Could you check a few things on this model? Use its own coordinates, in mm. A direction names the side the tool comes from. Round coordinates to 2 decimals unless told otherwise and drop trailing zeros. Loops run counter-clockwise (first coordinate to the right, second up) from the corner with the lowest first, then second, coordinate; pieces in that order, holes last. Notation, with made-up numbers: (10, 41) -> (51, 41) arc R27 ccw to (51, 80) -> close; hole circle Ø8 at (-19.5, 84.25). An arc over 180 degrees is marked (long way). Write each question's results on one line, items separated by ' | '. Start each with the question number.
1) Imagine slicing it at A-A, the plane x = 2.5. List the corners of the cut face in (y, z) for me.
2) For P1, Ø3, axis at y = 0, z = 2.5, coming from the +X side, with a flat end and sliding along its axis, tell me the tip position at first contact or that it passes through.
3) If I drill on probe 1 along X at (y, z) = (14.7, 0); probe 2 along Z at (x, y) = (2.5, 15.35); probe 3 along Y at (x, z) = (-1.75, 1.25), over which ranges is the centre line in solid material (lowest first)?
4) Which directions (+Z, -Z, +X, -X, +Y, -Y) give clear straight access to the entire face, cutting with the end or side of a thin tool? Please do faces 1 (the flat face through (0, 14, 0)), 2 (the cylindrical face through (0.35, -15.48, -0.09)).
5) We'd pull the mould along Z, two halves only. Please class faces 3 (the cylindrical face through (0.35, 15.52, -0.09)), 4 (the flat face through (6, 15, 0)), 5 (the flat face through (-3, 0, 5)): pulls with the +Z half, pulls with the -Z half, needs draft (parallel to the pull), parting line crosses it, or undercut.
6) Imagine slicing it at D-D, the plane z = 3.75. List the corners of the cut face in (x, y) for me, plus the area to 3 significant figures.
7) Imagine slicing it at C-C, the plane y = 15.5. List the corners of the cut face in (x, z) for me.
8) Imagine slicing it at B-B, the plane z = 0. List the corners of the cut face in (x, y) for me, plus the area to 3 significant figures.
from build123d import *

# Parameters (mm, degrees)
SKETCH1_W               = 12
SKETCH1_H               = 34
BOSS_EXTRUDE1_DEPTH     = 5
SKETCH2_W               = 16
SKETCH2_H               = 28
CUT_EXTRUDE1_DEPTH      = 1
CUT_EXTRUDE1_DEPTH_BACK = 11
SKETCH3_R               = 2.15
CUT_EXTRUDE2_DEPTH      = 35


with BuildPart() as part:
    # Sketch1 → Boss-Extrude1 (new body, symmetric)
    with BuildSketch(Plane.XY):
        Rectangle(SKETCH1_W, SKETCH1_H)
    extrude(amount=BOSS_EXTRUDE1_DEPTH, both=True)

    # Sketch2 → Cut-Extrude1 (cut, two sides)
    with BuildSketch(Plane.XY.offset(5)) as cut_extrude1_sk:
        with Locations((6, 0)):
            Rectangle(SKETCH2_W, SKETCH2_H)
    extrude(amount=CUT_EXTRUDE1_DEPTH, mode=Mode.SUBTRACT)
    extrude(cut_extrude1_sk.sketch, amount=-CUT_EXTRUDE1_DEPTH_BACK, mode=Mode.SUBTRACT)

    # Sketch3 → Cut-Extrude2 (cut, through all)
    with BuildSketch(Plane(origin=(0, 17, 0), x_dir=(1, 0, 0), z_dir=(0, 1, 0))):
        with Locations((2.5, 0)):
            Circle(SKETCH3_R)
    extrude(amount=-CUT_EXTRUDE2_DEPTH, mode=Mode.SUBTRACT)


solid = part.part
Checked values:
1) outline: (-17, -5) -> (-14, -5) -> (-14, -2.15) -> (-17, -2.15) -> close; (-17, 2.15) -> (-14, 2.15) -> (-14, 5) -> (-17, 5) -> close; (14, -5) -> (17, -5) -> (17, -2.15) -> (14, -2.15) -> close; (14, 2.15) -> (17, 2.15) -> (17, 5) -> (14, 5) -> close
2) P1: x = -2
3) probe 1: -6 to 0.35, 4.65 to 6 | probe 2: -5 to -2.15, 2.15 to 5 | probe 3: -17 to -14, 14 to 17
4) face 1: +Z, -Z, +X | face 2: +Y, -Y
5) face 3: undercut | face 4: needs draft | face 5: pulls with the +Z half
6) outline: (-6, -17) -> (6, -17) -> (6, -14) -> (-2, -14) -> (-2, 14) -> (6, 14) -> (6, 17) -> (-6, 17) -> close | area: 184 mm^2
7) outline: (-6, -5) -> (6, -5) -> (6, 5) -> (-6, 5) -> close; hole circle Ø4.3 at (2.5, 0)
8) outline: (-6, -17) -> (0.35, -17) -> (0.35, -14) -> (-2, -14) -> (-2, 14) -> (0.35, 14) -> (0.35, 17) -> (-6, 17) -> close; (4.65, -17) -> (6, -17) -> (6, -14) -> (4.65, -14) -> close; (4.65, 14) -> (6, 14) -> (6, 17) -> (4.65, 17) -> close | area: 158 mm^2
